Autodesk Inventor part; units mm, degrees
ref_plane "YZ Plane" through (0, 0, 0) normal (1, 0, 0) x (0, 1, 0)
ref_plane "XZ Plane" through (0, 0, 0) normal (0, 1, 0) x (-1, 0, 0)
ref_plane "XY Plane" through (0, 0, 0) normal (0, 0, 1) x (1, 0, 0)
sketch "Sketch1" plane through (0, 0, 0) normal (0, 0, 1) x (1, 0, 0)
  line L0 (0, 0) -> (76.2, 0)
  line L1 (76.2, 0) -> (76.2, 12.7)
  line L2 (0, 0) -> (0, 44.45)
  line L3 (0, 44.45) -> (12.7, 44.45)
  line L4 (12.7, 44.45) -> (12.7, 19.05)
  line L5 (12.7, 19.05) -> (38.1, 19.05)
  line L6 (38.1, 19.05) -> (38.1, 44.45)
  line L7 (38.1, 44.45) -> (50.8, 44.45)
  line L8 (50.8, 44.45) -> (50.8, 19.05)
  line L9 (57.15, 12.7) -> (76.2, 12.7)
  arc A0 (50.8, 19.05) -> (57.15, 12.7) centre (57.15, 19.05) ccw
  point P0 (50.8, 12.7)
  dimension "d1" = 12.7
  dimension "d2" = 44.45
  dimension "d3" = 12.7
  dimension "d6" = 12.7
  dimension "d7" = 76.2
  dimension "d8" = 50.8
  dimension "d9" = 19.05
  dimension "d28" = 6.35
extrude "Base" add sketch "Sketch1" along normal blind 50.8
sketch "Sketch2" plane through (50.8, 12.7, 0) normal (0, 1, 0) x (1, 0, 0)
  line L0 (25.4, 0) -> (25.4, -50.8)
  circle A0 centre (25.4, -25.4) radius 25.4
  point P0 (-50.8, 0)
extrude "Ciclre" add sketch "Sketch2" against normal blind 12.7
hole "Hole1" at (76.2, 0, 25.4) direction (0, 1, 0) diameter 19.05 end through all
sketch "Sketch4" plane through (50.8, 12.7, 0) normal (1, 0, 0) x (0, 0, -1)
  line L0 (-50.8, 31.75) -> (-38.1, 31.75)
  line L1 (0, 31.75) -> (-50.8, 31.75)
  line L2 (-38.1, 31.75) -> (-38.1, 12.7)
  line L3 (-38.1, 12.7) -> (-12.7, 12.7)
  line L4 (-12.7, 12.7) -> (-12.7, 31.75)
  line L5 (-38.1, 31.75) -> (-12.7, 31.75)
  line L6 (0, 31.75) -> (-50.8, 31.75)
  point P0 (0, -12.7)
  dimension "d23" = 12.7
  dimension "d24" = 19.05
  dimension "d25" = 25.4
extrude "Extrusion3" cut sketch "Sketch4" against normal through all
properties part number "tut" material "Titanium"
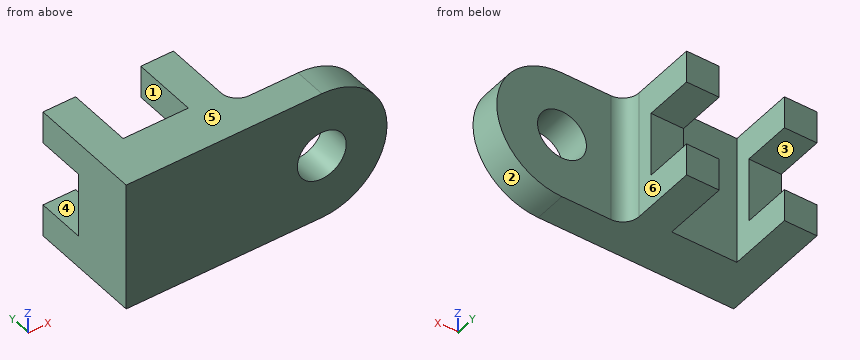
Read the model definition and answer for the solid it produces. Units are mm, in the model's axes. Face numbers are marked on the shaded views. A direction names the side the tool comes from. Round coordinates to 2 decimals unless told otherwise and drop trailing zeros. Write each loop counter-clockwise with the first axis right and the second up, starting at its lowest first coordinate (ties: lowest second). Pieces come first, ordered by that corner, then holes. Notation, with made-up numbers: (0.25, 48.25) - (37.25, 48.25) arc R19 cw to (37.25, 57.25) - close; hole circle Ø7 at (42.25, -8). An arc over 180 degrees is marked (long way). One line per question, with ' | ' between items. Start each with the question number.
1. For the marked faces 1, 2 and 3, determine the directions among +Z, -Z, +X, -X, +Y, -Y from which every point of the face is accessible in a straight line to the end or side of a thin tool.
2. Section B-B (z = 24.5) is taken. Determine the outline of the cut face in (x, y).
3. For a pull along Z with two mould halves and no side action, classify the marked faces 4, 5 and 6 as +Z half, -Z half, draft (parallel to the pull), parting line (faces both ways), or undercut.
4. Section C-C (x = 47) is taken. Determine the outline of the cut face in (y, z).
5. Find the intervals of material crossed by probe 1 along X at (y, z) = (3, 25); probe 2 along Z at (x, y) = (76.2, 8.5) (3 decimals); probe 3 along X at (y, z) = (21.5, 25.5), in increasing order. Write a range as [from, to].
6. Section A-A (y = 41) is taken. Determine the outline of the cut face in (x, z).
7. Section D-D (z = 14) is taken. Determine the outline of the cut face in (x, y), and give its area (3 significant figures).
8. Each of these flat-tipped pins is pushed along its axis until it touches: pin 1 (22 mm diameter, centred on x = 76.2, z = 25.4, fed in from +Y); pin 2 (8 mm diameter, centred on y = 24.5, z = 11, fed in from +X); pin 3 (20.5 mm diameter, centred on y = 28.5, z = 28.5, fed in from +X). Where does it stop, or does it pass through?
Filled in:
1) face 1: +Z, -Z, +Y | face 2: +X, +Y, -Y | face 3: +X, -X, +Y
2) outline: (0, 0) - (66.72, 0) - (66.72, 12.7) - (57.15, 12.7) arc R6.35 cw to (50.8, 19.05) - (50.8, 25.4) - (38.1, 25.4) - (38.1, 19.05) - (12.7, 19.05) - (12.7, 25.4) - (0, 25.4) - close; (85.68, 0) - (101.58, 0) - (101.58, 12.7) - (85.68, 12.7) - close
3) face 4: undercut | face 5: +Z half | face 6: draft
4) outline: (0, 0) - (44.45, 0) - (44.45, 12.7) - (25.4, 12.7) - (25.4, 38.1) - (44.45, 38.1) - (44.45, 50.8) - (0, 50.8) - close
5) probe 1: [0, 66.68], [85.72, 101.6] | probe 2: [0, 15.875], [34.925, 50.8] | probe 3: [0, 12.7], [38.1, 50.8]
6) outline: (0, 0) - (12.7, 0) - (12.7, 12.7) - (0, 12.7) - close; (0, 38.1) - (12.7, 38.1) - (12.7, 50.8) - (0, 50.8) - close; (38.1, 0) - (50.8, 0) - (50.8, 12.7) - (38.1, 12.7) - close; (38.1, 38.1) - (50.8, 38.1) - (50.8, 50.8) - (38.1, 50.8) - close
7) outline: (0, 0) - (98.9, 0) - (98.9, 12.7) - (57.15, 12.7) arc R6.35 cw to (50.8, 19.05) - (50.8, 25.4) - (38.1, 25.4) - (38.1, 19.05) - (12.7, 19.05) - (12.7, 25.4) - (0, 25.4) - close | area: 1,750 mm²
8) pin 1: y = 12.7 | pin 2: x = 50.8 | pin 3: x = 50.85
